Check sheet for the drawn part. Datum: minimum x, y, z corner. Units: mm. Give positions to 0.01 mm unless a question says otherwise; leave off trailing zeros. Order: outer loops, then holes, each group sorted by start corner. A loop starts at its lowest first (then second) coordinate and runs counter-clockwise, first axis right, second up. Notation, with made-up numbers: (-15, 63) -> (16, 63) arc R19 cw to (16, 92) -> close; hole circle Ø5 at (-2, 60.25). An arc over 180 degrees is marked (long way). Answer in a Markdown table with one row per item. Add a question column.
(1) Cross-section at B-B (y = 45). Record the cut outline in (x, z).
(2) Thickness scan on L1, parallel to Y at x = 212, z = 0.75; L2, parallel to X at y = 8, z = 1.35; L3, parallel to X at y = 57, z = 3.8. Record the ranges inside material, lowest first. Write a range as [from, to].
(3) Cross-section at A-A (z = 4.2). Record the cut outline in (x, y), then the cut area to 3 significant figures.
(4) Cross-section at C-C (x = 175). Record the cut outline in (y, z).
(5) Go/stop test with flat-tipped pins: pin 1 (1.6 mm diameter, centred on y = 3.5, z = 3, fed in from +X); pin 2 (1.5 mm diameter, centred on y = 64, z = 3.5, fed in from -X); pin 3 (1.6 mm diameter, centred on x = 216.5, z = 3.5, fed in from -Y). Record where each tip stops, or that it passes through.
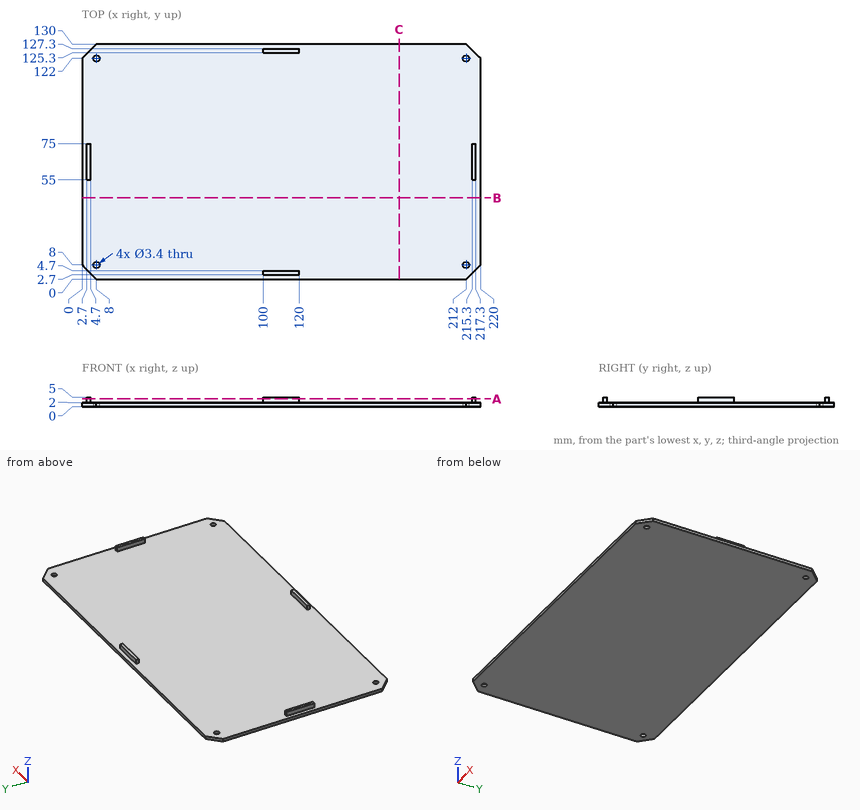
Answer below:
| question | item | result |
|---|---|---|
| 1 | outline | (0, 0) -> (220, 0) -> (220, 2) -> (0, 2) -> close |
| 2 | L1 | y = [0, 6.3], [9.7, 120.3], [123.7, 130] |
| 2 | L2 | x = [0, 6.3], [9.7, 210.3], [213.7, 220] |
| 2 | L3 | x = [2.7, 4.7], [215.3, 217.3] |
| 3 | outline | (2.7, 55) -> (4.7, 55) -> (4.7, 75) -> (2.7, 75) -> close; (100, 2.7) -> (120, 2.7) -> (120, 4.7) -> (100, 4.7) -> close; (100, 125.3) -> (120, 125.3) -> (120, 127.3) -> (100, 127.3) -> close; (215.3, 55) -> (217.3, 55) -> (217.3, 75) -> (215.3, 75) -> close |
| 3 | area | 160 mm² |
| 4 | outline | (0, 0) -> (130, 0) -> (130, 2) -> (0, 2) -> close |
| 5 | pin 1 | stops at x = 120 |
| 5 | pin 2 | stops at x = 2.7 |
| 5 | pin 3 | stops at y = 55 |
